Read the model definition and answer for the solid it produces. Units are mm, in the model's axes. Face numbers are marked on the shaded views. A direction names the side the tool comes from. Coordinates: 2 decimals unless noted, no trailing zeros. Loops run counter-clockwise (first coordinate to the right, second up) from the corner with the lowest first, then second, coordinate; pieces in that order, holes last. Notation, with made-up numbers: M -15.5,14.25 L 13.5,14.25 A24 ccw 13.5,49.25 Z; hole C 72,-28 d6. An arc over 180 degrees is marked long. Put each result on its own line as item: value.
from build123d import *

# Parameters (mm, degrees)
SKETCH1_W                            = 400
SKETCH1_H                            = 114
BASE_FLANGE1_DEPTH                   = 1
EDGE_FLANGE1_STRIP_W                 = 10
EDGE_FLANGE1_STRIP_H                 = 1
EDGE_FLANGE1_STRIP_CUT_DEPTH         = 400
EDGE_FLANGE1_DEPTH                   = 400
F_4_2_START                          = -57
F_4_2_4_2_DIAMETER_HOLE1_OUTLINE_R   = 2.1
F_4_2_4_2_DIAMETER_HOLE1_DEPTH       = 1
F_4_2_START_2                        = -1
F_4_2_4_2_DIAMETER_HOLE1_2_OUTLINE_R = 2.1
F_4_2_4_2_DIAMETER_HOLE1_2_DEPTH     = 1


# Read off the part's stored shape, not the designer's step: Ø4.2 (4.2) Diameter Hole1
# Sheet-metal steps are written as plain solids
with BuildPart() as part:
    # Sketch1 → Base-Flange1 (new body)
    with BuildSketch(Plane(origin=(0, 0, 0), x_dir=(0, 0, -1), z_dir=(1, 0, 0))):
        Rectangle(SKETCH1_W, SKETCH1_H)
    extrude(amount=-BASE_FLANGE1_DEPTH)

    # Edge-Flange1 strip (across the edge) → Edge-Flange1 strip cut (cut)
    with BuildSketch(Plane(origin=(0, -57, 200), x_dir=(0, 1, 0), z_dir=(0, 0, -1))):
        with Locations((-1, -0.5)):
            Rectangle(EDGE_FLANGE1_STRIP_W, EDGE_FLANGE1_STRIP_H)
    extrude(amount=EDGE_FLANGE1_STRIP_CUT_DEPTH, mode=Mode.SUBTRACT)

    # Edge-Flange1 section (across the edge) → Edge-Flange1 (add)
    with BuildSketch(Plane(origin=(0, -57, 200), x_dir=(0, 1, 0), z_dir=(0, 0, -1))):
        with BuildLine():
            Line((0, 3), (0, 324))
            Line((0, 324), (1, 324))
            Line((1, 324), (1, 3))
            ThreePointArc((1, 3), (1.878679656, 0.878679656), (4, 0))
            Line((4, 0), (4, -1))
            ThreePointArc((4, -1), (1.171572875, 0.171572875), (0, 3))
        make_face()
    extrude(amount=EDGE_FLANGE1_DEPTH)

    # Ø4.2 (4.2) Diameter Hole1 outline → Ø4.2 (4.2) Diameter Hole1 (cut)
    with BuildSketch(Plane(origin=(0, 0, 0), x_dir=(1, 0, 0), z_dir=(0, 1, 0)).offset(F_4_2_START)):
        with Locations((15, 160)):
            Circle(F_4_2_4_2_DIAMETER_HOLE1_OUTLINE_R)
        with Locations((15, 0)):
            Circle(F_4_2_4_2_DIAMETER_HOLE1_OUTLINE_R)
        with Locations((15, -160)):
            Circle(F_4_2_4_2_DIAMETER_HOLE1_OUTLINE_R)
        with Locations((316.678974837, -160)):
            Circle(F_4_2_4_2_DIAMETER_HOLE1_OUTLINE_R)
        with Locations((316.678974837, 0)):
            Circle(F_4_2_4_2_DIAMETER_HOLE1_OUTLINE_R)
        with Locations((316.678974837, 160)):
            Circle(F_4_2_4_2_DIAMETER_HOLE1_OUTLINE_R)
    extrude(amount=F_4_2_4_2_DIAMETER_HOLE1_DEPTH, mode=Mode.SUBTRACT)

    # 4.2 _4.2_ Diameter Hole1 2 outline → 4.2 _4.2_ Diameter Hole1 2 (cut)
    with BuildSketch(Plane.YZ.offset(F_4_2_START_2)):
        with Locations((42, -160)):
            Circle(F_4_2_4_2_DIAMETER_HOLE1_2_OUTLINE_R)
        with Locations((42, 0)):
            Circle(F_4_2_4_2_DIAMETER_HOLE1_2_OUTLINE_R)
        with Locations((42, 160)):
            Circle(F_4_2_4_2_DIAMETER_HOLE1_2_OUTLINE_R)
        with Locations((-41, 160)):
            Circle(F_4_2_4_2_DIAMETER_HOLE1_2_OUTLINE_R)
        with Locations((-41, 0)):
            Circle(F_4_2_4_2_DIAMETER_HOLE1_2_OUTLINE_R)
        with Locations((-41, -160)):
            Circle(F_4_2_4_2_DIAMETER_HOLE1_2_OUTLINE_R)
    extrude(amount=F_4_2_4_2_DIAMETER_HOLE1_2_DEPTH, mode=Mode.SUBTRACT)


solid = part.part
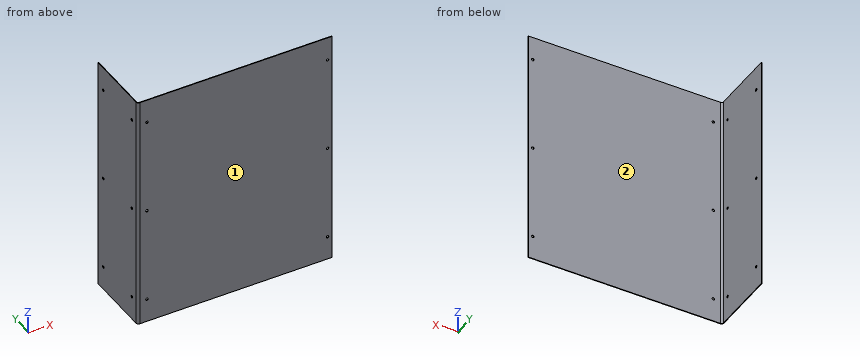
1) Find section C-C, the plane y = 5. Write down the section's boundary in (x, z), plus the area to 3 significant figures.
Answer list:
outline: M -1,-200 L 0,-200 L 0,200 L -1,200 Z
area: 400 mm^2
2) Which of the six approach directions +Z, -Z, +X, -X, +Y, -Y give full straight-line access (tool end or side, diameter ignored) to the marked faces 1 and 2?
Answer list:
face 1: +Z, -Z, +X, -X, -Y
face 2: +Z, -Z, +X, +Y
3) Given pin 1 Ø2.5 at (x, z) = (15, 160) entering from +Y; pin 2 Ø5 at (y, z) = (-41, -160) entering from -X; pin 3 Ø5.5 at (y, z) = (-41, 160) entering from +X; pin 4 Ø1 at (x, z) = (111, 2) entering from +Y, each flat-ended and moving along its own axis, determine where each tip first touches the part or whether it passes through.
Answer list:
pin 1: passes through
pin 2: stops at x = -1
pin 3: stops at x = 0
pin 4: stops at y = -56
4) Find section A-A, the plane z = -94.5. Write down the section's boundary in (x, y), plus the area to 3 significant figures.
Answer list:
outline: M -1,-53 A4 ccw 3,-57 L 324,-57 L 324,-56 L 3,-56 A3 cw 0,-53 L 0,57 L -1,57 Z
area: 436 mm^2
5) Straight lines are drawn through the part: line 1 (Y direction, x = 139, z = 87.5); line 2 (X direction, y = 24.5, z = -71). For each, find the intervals that lie inside material, in ascending order. Write a range as [from, to].
Answer list:
line 1: y = [-57, -56]
line 2: x = [-1, 0]
6) Find section B-B, the plane x = 33.5. Write down the section's boundary in (y, z).
Answer list:
outline: M -57,-200 L -56,-200 L -56,200 L -57,200 Z
